Could you check a few things on this model? Use its own coordinates, in mm. Face numbers are marked on the shaded views. A direction names the side the tool comes from. Give positions to 0.01 mm unless a question says otherwise; leave off trailing zeros. Loops run counter-clockwise (first coordinate to the right, second up) from the corner with the lowest first, then second, coordinate; pieces in that order, holes last. Notation, with made-up numbers: (51.25, -5.5) - (75.25, -5.5) arc R22 cw to (75.25, 9.5) - close; hole circle Ø4 at (56, 49). An arc over 180 degrees is marked (long way). Answer in a Markdown table with one row per item. Add a question column.
```python
from build123d import *

# Parameters (mm, degrees)
SKETCH_3_R               = 6.5
SKETCH_3_R_2             = 5.1
EXTRUDE_1_DEPTH          = 20
EXTRUDE_START            = -18.7999999
EXTRUDE_2_OUTLINE_R      = 9.5
EXTRUDE_2_DEPTH          = 18.7999999
EXTRUDE_START_2          = -31.801
EXTRUDE_2_2_OUTLINE_R    = 9.5
EXTRUDE_2_2_DEPTH        = 0.0009999
EXTRUDE_START_3          = -31.8000001
EXTRUDE_2_3_OUTLINE_R    = 9.5
EXTRUDE_2_3_DEPTH        = 13.0000002
EXTRUDE_START_4          = -9.5000001
EXTRUDE_2_4_OUTLINE_R    = 6.5
EXTRUDE_2_4_DEPTH        = 19.5000001
CUT_EXTRUDE_1_DEPTH      = 39.749885281
CUT_EXTRUDE_1_DEPTH_BACK = 39.749885281
CUT_EXTRUDE_2_DEPTH      = 39.749064529
CUT_EXTRUDE_2_DEPTH_BACK = 39.749064529
SHELL_1_T                = -1.5
FILLET_1_R               = 0.6
EXTRUDE_START_5          = 6
SKETCH_6_W               = 4.8
SKETCH_6_H               = 6
SKETCH_6_R               = 1.5
EXTRUDE_3_DEPTH          = 1.729857
CUT_EXTRUDE_3_DEPTH      = 39.749064611
CUT_EXTRUDE_3_DEPTH_BACK = 39.749064611
SKETCH_6_2_R             = 1.5
CUT_EXTRUDE_START        = 9.5
CUT_EXTRUDE_4_DEPTH      = 2.5
CUT_EXTRUDE_START_2      = -9.5
SKETCH_8_R               = 2.5
CUT_EXTRUDE_5_DEPTH      = 1


with BuildPart() as part:
    # Sketch 3 → Extrude 1 (new, symmetric)
    with BuildSketch(Plane(origin=(0, 0, 0), x_dir=(0, 0, -1), z_dir=(1, 0, 0))):
        with Locations((25.3, 0)):
            Circle(SKETCH_3_R)
        with Locations((25.3, 0)):
            Circle(SKETCH_3_R_2, mode=Mode.SUBTRACT)
    extrude(amount=EXTRUDE_1_DEPTH, both=True)

    # Fillet 1
    fillet_1_edges = [part.edges().sort_by_distance(p)[0] for p in [
        (-20, 0, -18.8),
        (20, 0, -18.8),
    ]]
    fillet(fillet_1_edges, radius=FILLET_1_R)



with BuildPart() as body_2:
    # Extrude 2: read off the stored shape, not the designer's step
    # Extrude 2 outline → Extrude 2 (new body)
    with BuildSketch(Plane.XY.offset(EXTRUDE_START)):
        Circle(EXTRUDE_2_OUTLINE_R)
    extrude(amount=EXTRUDE_2_DEPTH)

    # Extrude 2 2 outline → Extrude 2 2 (add)
    with BuildSketch(Plane.XY.offset(EXTRUDE_START_2)):
        Circle(EXTRUDE_2_2_OUTLINE_R)
    extrude(amount=EXTRUDE_2_2_DEPTH)

    # Extrude 2 3 outline → Extrude 2 3 (add)
    with BuildSketch(Plane.XY.offset(EXTRUDE_START_3)):
        Circle(EXTRUDE_2_3_OUTLINE_R)
    extrude(amount=EXTRUDE_2_3_DEPTH)

    # Extrude 2 4 outline → Extrude 2 4 (cut)
    with BuildSketch(Plane.YZ.offset(EXTRUDE_START_4)):
        with Locations((0, -25.3)):
            Circle(EXTRUDE_2_4_OUTLINE_R)
    extrude(amount=EXTRUDE_2_4_DEPTH, mode=Mode.SUBTRACT)

    # Sketch 4 → Cut-Extrude 1 (cut, two sides: drawn at the far end of the back side and taken through both)
    with BuildSketch(Plane(origin=(0, 0, 0), x_dir=(0, 0, -1), z_dir=(1, 0, 0)).offset(-CUT_EXTRUDE_1_DEPTH_BACK)):
        with BuildLine():
            Line((25.3, -12.675131419), (25.3, -6.5))
            ThreePointArc((25.3, -6.5), (31.8, 0), (25.3, 6.5))
            Line((25.3, 6.5), (25.3, 12.675131419))
            ThreePointArc((25.3, 12.675131419), (37.975131419, 0), (25.3, -12.675131419))
        make_face()
    extrude(amount=CUT_EXTRUDE_1_DEPTH + CUT_EXTRUDE_1_DEPTH_BACK, mode=Mode.SUBTRACT)

    # Sketch 5 → Cut-Extrude 2 (cut, two sides: drawn at the far end of the back side and taken through both)
    with BuildSketch(Plane(origin=(0, 0, 0), x_dir=(0, 0, -1), z_dir=(1, 0, 0)).offset(-CUT_EXTRUDE_2_DEPTH_BACK)):
        Polygon((26.434429002, 6.400239905), (13, 9.5), (13, 10.602524511), (26.434429002, 10.602524511), align=None)
        Polygon((13, -10.602524511), (13, -9.5), (26.434429002, -6.400239905), (26.434429002, -10.602524511), align=None)
    extrude(amount=CUT_EXTRUDE_2_DEPTH + CUT_EXTRUDE_2_DEPTH_BACK, mode=Mode.SUBTRACT)

    # Shell 1
    shell_1_openings = [body_2.faces().sort_by_distance(p)[0] for p in [
        (0, 0, 0),
    ]]
    offset(amount=SHELL_1_T, openings=shell_1_openings)


with BuildPart() as part_1:
    add(part.part)

    add(body_2.part)  # Extrude 3 merges body 2
    # Sketch 6 → Extrude 3 (add)
    with BuildSketch(Plane(origin=(0, 0, 0), x_dir=(0, 0, -1), z_dir=(0, 1, 0)).offset(EXTRUDE_START_5)):
        with Locations((16.4, 0)):
            Rectangle(SKETCH_6_W, SKETCH_6_H)
        with Locations((16.4, 0)):
            Circle(SKETCH_6_R, mode=Mode.SUBTRACT)
    extrude_3 = extrude(amount=EXTRUDE_3_DEPTH)

    # Mirror 1: Extrude 3 across plane
    add(extrude_3.mirror(Plane.ZX))

    # Sketch 6_2 → Cut-Extrude 3 (cut, two sides: drawn at the far end of the back side and taken through both)
    with BuildSketch(Plane(origin=(0, 0, 0), x_dir=(0, 0, -1), z_dir=(0, 1, 0)).offset(-CUT_EXTRUDE_3_DEPTH_BACK)):
        with Locations(Location((16.4, 0, 0), (0, 0, 180))):
            Circle(SKETCH_6_2_R)
    extrude(amount=CUT_EXTRUDE_3_DEPTH + CUT_EXTRUDE_3_DEPTH_BACK, mode=Mode.SUBTRACT)

    # Sketch 7 → Cut-Extrude 4 (cut)
    with BuildSketch(Plane(origin=(0, 0, 0), x_dir=(1, 0, 0), z_dir=(0, 1, 0)).offset(CUT_EXTRUDE_START)):
        Polygon((3.290896534, 16.4), (1.645448267, 19.25), (-1.645448267, 19.25), (-3.290896534, 16.4), (-1.645448267, 13.55), (1.645448267, 13.55), align=None)
    extrude(amount=-CUT_EXTRUDE_4_DEPTH, mode=Mode.SUBTRACT)

    # Sketch 8 → Cut-Extrude 5 (cut)
    with BuildSketch(Plane(origin=(0, 0, 0), x_dir=(1, 0, 0), z_dir=(0, 1, 0)).offset(CUT_EXTRUDE_START_2)):
        with Locations((0, 16.4)):
            Circle(SKETCH_8_R)
    extrude(amount=CUT_EXTRUDE_5_DEPTH, mode=Mode.SUBTRACT)


solid = part_1.part
```
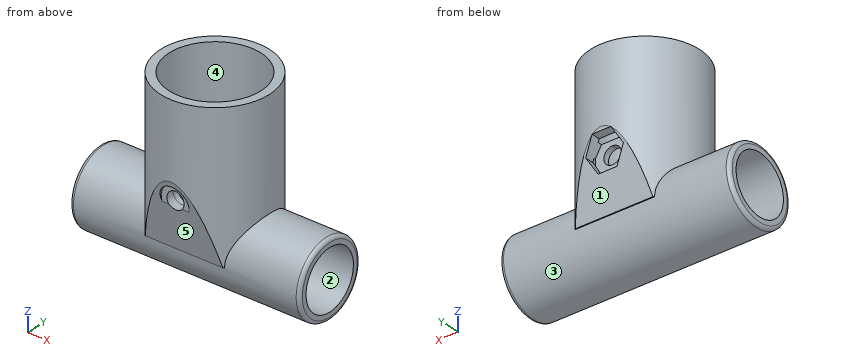
(1) For pin 1 Ø1.4 at (x, y) = (1.5, -6.5) entering from +Z; pin 2 Ø6.5 at (x, z) = (0, -16.4) entering from +Y; pin 3 Ø1.1 at (y, z) = (-6.5, -17.5) entering from +X, each with a flat end and sliding along its axis, tell me the tip position at first contact or that it passes through.
(2) I want a section at A-A on y = 0. Please give me the cut outline in (x, z).
(3) On a 3-axis mill with a long thin cutter (end or side, diameter ignored), from which of +Z, -Z, +X, -X, +Y, -Y can I reach the whole of each face in a straight line? I mean the marked faces 4 and 5. Say none if no direction works.
(4) I want a section at B-B on x = -11. Please give me the cut outline in (y, z).
(5) Please list where these lines run through material, in increasing order: line 1 (Y direction, x = 0, z = -3.5); line 2 (Z direction, x = -6, y = -1.25).
(6) We'd pull the mould along Z, two halves only. Please class the marked faces 1, 2 and 3: pulls with the +Z half, pulls with the -Z half, needs draft (parallel to the pull), parting line crosses it, or undercut.
Reported:
| question | item | result |
|---|---|---|
| 1 | pin 1 | z = -14 |
| 1 | pin 2 | y = 9.47 |
| 1 | pin 3 | x = 7.41 |
| 2 | outline | (-20, -31.2) arc R0.6 ccw to (-19.4, -31.8) - (19.4, -31.8) arc R0.6 ccw to (20, -31.2) - (20, -30.4) - (-20, -30.4) - close; (-20, -20.2) - (20, -20.2) - (20, -19.4) arc R0.6 ccw to (19.4, -18.8) - (9.5, -18.8) - (9.5, 0) - (8, 0) - (8, -17.3) - (1.2, -17.3) arc R1.5 cw to (-1.2, -17.3) - (-8, -17.3) - (-8, 0) - (-9.5, 0) - (-9.5, -18.8) - (-19.4, -18.8) arc R0.6 ccw to (-20, -19.4) - close |
| 3 | face 4 | +Z |
| 3 | face 5 | -Z, +X, -X, -Y |
| 4 | outline | circle Ø13 at (0, -25.3); hole circle Ø10.2 at (0, -25.3) |
| 5 | line 1 | -9.5 to -8, 8 to 9.5 |
| 5 | line 2 | -31.68 to -30.24, -20.36 to -17.4 |
| 6 | face 1 | pulls with the -Z half |
| 6 | face 2 | undercut |
| 6 | face 3 | parting line crosses it |
